Geometry: final body of the model. Coordinates: model frame, mm. A direction names the side the tool comes from. Give positions to 0.01 mm unless a question says otherwise; leave off trailing zeros. Write each loop counter-clockwise with the first axis right and the second up, starting at its lowest first coordinate (ties: lowest second). Pieces come first, ordered by that corner, then holes. Notation, with made-up numbers: M -12.5,66 L 9.5,66 A30 cw 9.5,100 Z; hole C -33.5,37.5 d3. An arc over 180 degrees is marked long. Use a Markdown table: item, result. Add a question column.
(1) Material intervals for L1, parallel to Y at x = 321, z = 39; L2, parallel to Y at x = 238, z = 86.5; L3, parallel to Y at x = 252.5, z = 148.5, sorted ascending.
(2) Cut plane D-D (y = 327). Output: boundary loops of the cut face in (x, z), plus the area to 3 significant figures.
(3) Cut plane A-A (z = 181.5). Output: boundary loops of the cut face in (x, y), plus the area to 3 significant figures.
(4) Pin query (flat end, axial travel): pin 1 Ø3 at (x, z) = (392.5, 89.5) entering from -Y; pin 2 Ø12 at (y, z) = (276.5, 104.5) entering from +X; pin 3 Ø6 at (x, z) = (121.5, 87.5) entering from +Y. Return the tip coordinate at first contact, or that it passes through.
(5) Reachability of faces 5 (the flat face through (222.8, 304.1, 102.5)), 6 (the flat face through (305.157, 258.793, 102.544)), 7 (the flat face through (97.885, 81.778, 102.544)), 8 (the flat face through (154.126, 43, 103)) from +Z, -Z, +X, -X, +Y, -Y: full face, straight path, thin tool, end or side. Return the list, or none.
(6) Draft query along X for faces 1 (the flat face through (136.579, 165.148, 102.544)), 2 (the flat face through (216, 185, 0)), 3 (the flat face through (336.729, 8, 103)), 4 (the flat face through (204.17, 300.3, 102.54)). Return one class per face: released by +X, released by -X, zero draft, split by the parting line, or undercut.
(7) Cut plane B-B (y = 89.5). Output: boundary loops of the cut face in (x, z).
(8) Cut plane C-C (x = 360.5). Output: boundary loops of the cut face in (y, z), plus the area to 3 significant figures.
```python
from build123d import *

# Parameters (mm, degrees)
SKETCH_1_R      = 99.790649717
SKETCH_1_R_2    = 99.803620069
EXTRUDE_1_DEPTH = 208


with BuildPart() as part:
    # 草图1 → 凸台-拉伸1 (new body)
    with BuildSketch(Plane.XY):
        with Locations((100.652828051, 264.261906095)):
            Circle(SKETCH_1_R)
        with BuildLine():
            Line((51.162061057, 0), (336.729475208, 3.724305137))
            Line((336.729475208, 3.724305137), (336.729475208, 12.826055388))
            Line((336.729475208, 12.826055388), (154.125610781, 33.873852846))
            Line((154.125610781, 33.873852846), (154.125610781, 51.508493959))
            Line((154.125610781, 51.508493959), (191.67033057, 137.40626196))
            Line((191.67033057, 137.40626196), (240.662425477, 110.352897381))
            ThreePointArc((240.662425477, 110.352897381), (253.352736169, 192.261361688), (323.548842254, 236.335698903))
            Line((323.548842254, 236.335698903), (299.418472532, 248.397124418))
            Line((299.418472532, 248.397124418), (311.058094029, 269.483395245))
            Line((311.058094029, 269.483395245), (296.467383181, 277.537467633))
            Line((296.467383181, 277.537467633), (301.706884634, 286.436303433))
            Line((301.706884634, 286.436303433), (292.477329355, 291.87052757))
            Line((292.477329355, 291.87052757), (287.237827902, 282.971691769))
            Line((287.237827902, 282.971691769), (249.158038274, 302.482086968))
            Line((249.158038274, 302.482086968), (254.098559787, 311.432307098))
            Line((254.098559787, 311.432307098), (244.217516762, 316.886642848))
            Line((244.217516762, 316.886642848), (239.358147451, 308.083437573))
            Line((239.358147451, 308.083437573), (228.350833321, 314.159474973))
            Line((228.350833321, 314.159474973), (217.125127284, 293.823050994))
            Line((217.125127284, 293.823050994), (190.848647814, 306.957197033))
            ThreePointArc((190.848647814, 306.957197033), (198.015226406, 286.14196911), (200.443477768, 264.261906095))
            ThreePointArc((200.443477768, 264.261906095), (180.931523877, 204.987082034), (130.025963153, 168.892137797))
            Line((130.025963153, 168.892137797), (143.317282357, 161.298356371))
            Line((143.317282357, 161.298356371), (51.162061057, 0))
        make_face()
        with Locations((336.729475208, 137.40626196)):
            Circle(SKETCH_1_R_2)
    extrude(amount=EXTRUDE_1_DEPTH)


solid = part.part
```
Answer list:
| question | item | result |
|---|---|---|
| 1 | L1 | 3.52 to 14.64, 38.85 to 237.61 |
| 1 | L2 | 2.44 to 24.21, 111.82 to 308.83 |
| 1 | L3 | 2.63 to 22.53, 83.87 to 300.77, 308.54 to 312.31 |
| 2 | outline | M 23.05,0 L 178.26,0 L 178.26,208 L 23.05,208 Z |
| 2 | area | 32,300 mm² |
| 3 | outline | M 51.16,0 L 336.73,3.72 L 336.73,12.83 L 154.13,33.87 L 154.13,51.51 L 191.67,137.41 L 240.66,110.35 A99.8 ccw long 323.55,236.34 L 299.42,248.4 L 311.06,269.48 L 296.47,277.54 L 301.71,286.44 L 292.48,291.87 L 287.24,282.97 L 249.16,302.48 L 254.1,311.43 L 244.22,316.89 L 239.36,308.08 L 228.35,314.16 L 217.13,293.82 L 190.85,306.96 A99.79 ccw long 130.03,168.89 L 143.32,161.3 Z |
| 3 | area | 93,300 mm² |
| 4 | pin 1 | y = 53.65 |
| 4 | pin 2 | x = 309.22 |
| 4 | pin 3 | y = 362.44 |
| 5 | face 5 | +Z, -Z, +Y |
| 5 | face 6 | +Z, -Z, +X |
| 5 | face 7 | +Z, -Z, -X |
| 5 | face 8 | +Z, -Z |
| 6 | face 1 | undercut |
| 6 | face 2 | zero draft |
| 6 | face 3 | released by +X |
| 6 | face 4 | undercut |
| 7 | outline | M 102.3,0 L 170.73,0 L 170.73,208 L 102.3,208 Z; M 249.18,0 L 424.28,0 L 424.28,208 L 249.18,208 Z |
| 8 | outline | M 40.47,0 L 234.34,0 L 234.34,208 L 40.47,208 Z |
| 8 | area | 40,300 mm² |
